Here's how the part is built. I have some questions about the finished solid (model axes, mm). A direction names the side the tool comes from. Coordinates: 2 decimals unless noted, no trailing zeros. Loops run counter-clockwise (first coordinate to the right, second up) from the corner with the lowest first, then second, coordinate; pieces in that order, holes last. Notation, with made-up numbers: (-40, -2) -> (9, -2) arc R11 cw to (9, 8) -> close; hole circle Ø8 at (49.25, 24.25). An arc over 180 degrees is marked (long way). Answer as a JSON object with one key per item and string values. Group by question number.
1) I'm going to push flat-ended pins straight in: pin 1 (3 mm diameter, centred on x = 21, z = 23, fed in from -Y); pin 2 (15 mm diameter, centred on x = 11, z = 29, fed in from +Y); pin 3 (1 mm diameter, centred on x = 14.5, z = 43.5, fed in from +Y); pin 4 (4 mm diameter, centred on x = 32.5, y = 19, fed in from +Z). Where does each tip first touch, or does it pass through?
2) Which directions (+Z, -Z, +X, -X, +Y, -Y) give clear straight access to the entire face, cutting with the end or side of a thin tool? Please do faces 1 (the flat face through (29, 18, 20)), 2 (the flat face through (10, 5, 40)), 3 (the flat face through (20, 0, 25)).
3) I want a section at B-B (y = 4). Write out the boundary of the cut face in (x, z), then the cut area to 3 significant figures.
4) I want a section at C-C (z = 5). Write out the boundary of the cut face in (x, y).
5) I need wall thicknesses on probe 1 along Y at (x, z) = (35, 34.5); probe 2 along Z at (x, y) = (37, 31); probe 3 along Y at (x, z) = (28, 7.5). Which ranges of each line are inside material? Lowest first, please. Write a range as [from, to].
6) I want a section at D-D (y = 27). Write out the boundary of the cut face in (x, z), then the cut area to 3 significant figures.
7) I want a section at A-A (z = 37). Write out the boundary of the cut face in (x, y), then the cut area to 3 significant figures.
```python
from build123d import *

# Parameters (mm, degrees)
BOSS_EXTRUDE1_DEPTH = 20
SKETCH3_W           = 40
SKETCH3_H           = 10
BOSS_EXTRUDE2_DEPTH = 30
CUT_EXTRUDE2_DEPTH  = 20


with BuildPart() as part:
    # Sketch1 → Boss-Extrude1 (new body)
    with BuildSketch(Plane.XY):
        Polygon((0, 10), (40, 37.966903073), (40, 10), (40, 0), (0, 0), align=None)
    extrude(amount=BOSS_EXTRUDE1_DEPTH)

    # Sketch3 → Boss-Extrude2 (add)
    with BuildSketch(Plane.XY.offset(20)):
        with Locations((20, 5)):
            Rectangle(SKETCH3_W, SKETCH3_H)
    extrude(amount=BOSS_EXTRUDE2_DEPTH)

    # Sketch4 → Cut-Extrude2 (cut)
    with BuildSketch(Plane.ZY):
        Polygon((50, 10), (30, 10), (50, 0), align=None)
    extrude(amount=-CUT_EXTRUDE2_DEPTH, mode=Mode.SUBTRACT)


solid = part.part
```
Determined:
{
 "1": {"pin 1": "y = 0", "pin 2": "y = 10", "pin 3": "y = 3.5", "pin 4": "z = 20"},
 "2": {"face 1": "+Z, +X, -X, +Y", "face 2": "+Z, -X, +Y", "face 3": "+Z, -Z, +X, -X, -Y"},
 "3": {"outline": "(0, 0) -> (40, 0) -> (40, 50) -> (20, 50) -> (20, 42) -> (0, 42) -> close", "area": "1,840 mm^2"},
 "4": {"outline": "(0, 0) -> (40, 0) -> (40, 37.97) -> (0, 10) -> close"},
 "5": {"probe 1": "[0, 10]", "probe 2": "[0, 20]", "probe 3": "[0, 29.58]"},
 "6": {"outline": "(24.31, 0) -> (40, 0) -> (40, 20) -> (24.31, 20) -> close", "area": "314 mm^2"},
 "7": {"outline": "(0, 0) -> (40, 0) -> (40, 10) -> (20, 10) -> (20, 6.5) -> (0, 6.5) -> close", "area": "330 mm^2"}
}
